from build123d import *

# Parameters (mm, degrees)
SKETCH2_W                      = 500
SKETCH2_H                      = 30
BOSS_EXTRUDE1_DEPTH            = 10
CONVERT_SOLID1_START           = -500
CONVERT_SOLID1_DEPTH           = 497
CONVERT_SOLID1_START_2         = -3.414213562
CONVERT_SOLID1_2_DEPTH         = 3.414213562
CONVERT_SOLID1_START_3         = -3.5
CONVERT_SOLID1_3_DEPTH         = 0.085786438
CONVERT_SOLID1_START_4         = 290.130873959
CONVERT_SOLID1_4_DEPTH         = 23.171572876
EDGE_FLANGE1_STRIP_W           = 10
EDGE_FLANGE1_STRIP_H           = 2
EDGE_FLANGE1_STRIP_CUT_DEPTH   = 496.585786438
EDGE_FLANGE1_STRIP_2_W         = 10
EDGE_FLANGE1_STRIP_2_H         = 2
EDGE_FLANGE1_STRIP_CUT_2_DEPTH = 496.585786438
EDGE_FLANGE1_DEPTH             = 496.585786438
EDGE_FLANGE1_BEND_DEPTH        = 496.585786438
CUT_EXTRUDE1_DEPTH             = 592.923511083
CUT_EXTRUDE1_DEPTH_BACK        = 592.923511083
SKETCH43_R                     = 3


with BuildPart() as part:
    # Sketch2 → Boss-Extrude1 (new body)
    with BuildSketch(Plane.XY):
        with Locations((-250, 301.716660397)):
            Rectangle(SKETCH2_W, SKETCH2_H)
    extrude(amount=BOSS_EXTRUDE1_DEPTH)

    # Convert-Solid1: read off the stored shape, not the designer's step
    # Convert-Solid1 outline → Convert-Solid1 (cut)
    with BuildSketch(Plane.YZ.offset(CONVERT_SOLID1_START)):
        with BuildLine():
            Line((314.716660397, 3), (314.716660397, 10))
            Line((314.716660397, 10), (288.716660397, 10))
            Line((288.716660397, 10), (288.716660397, 3))
            ThreePointArc((288.716660397, 3), (289.009553616, 2.292893219), (289.716660397, 2))
            Line((289.716660397, 2), (313.716660397, 2))
            ThreePointArc((313.716660397, 2), (314.423767178, 2.292893219), (314.716660397, 3))
        make_face()
        with BuildLine():
            Line((316.716660397, 0), (316.716660397, 3))
            ThreePointArc((316.716660397, 3), (315.837980741, 0.878679656), (313.716660397, 0))
            Line((313.716660397, 0), (316.716660397, 0))
        make_face()
        with BuildLine():
            Line((286.716660397, 0), (289.716660397, 0))
            ThreePointArc((289.716660397, 0), (287.595340053, 0.878679656), (286.716660397, 3))
            Line((286.716660397, 3), (286.716660397, 0))
        make_face()
    extrude(amount=CONVERT_SOLID1_DEPTH, mode=Mode.SUBTRACT)

    # Convert-Solid1 2 outline → Convert-Solid1 2 (cut)
    with BuildSketch(Plane.YZ.offset(CONVERT_SOLID1_START_2)):
        Polygon((316.716660397, 10), (313.302446835, 10), (313.302446835, 3.5), (313.216660397, 3.5), (313.216660397, 0), (316.716660397, 0), align=None)
        Polygon((290.130873959, 3.5), (290.130873959, 10), (286.716660397, 10), (286.716660397, 0), (290.216660397, 0), (290.216660397, 3.5), align=None)
    extrude(amount=CONVERT_SOLID1_2_DEPTH, mode=Mode.SUBTRACT)

    # Convert-Solid1 3 outline → Convert-Solid1 3 (cut)
    with BuildSketch(Plane.YZ.offset(CONVERT_SOLID1_START_3)):
        with BuildLine():
            Line((316.716660397, 3.5), (314.716660397, 3.5))
            Line((314.716660397, 3.5), (314.716660397, 3))
            ThreePointArc((314.716660397, 3), (314.423767178, 2.292893219), (313.716660397, 2))
            Line((313.716660397, 2), (313.216660397, 2))
            Line((313.216660397, 2), (313.216660397, 0))
            Line((313.216660397, 0), (313.716660397, 0))
            ThreePointArc((313.716660397, 0), (315.837980741, 0.878679656), (316.716660397, 3))
            Line((316.716660397, 3), (316.716660397, 3.5))
        make_face()
        with BuildLine():
            Line((290.216660397, 0), (290.216660397, 2))
            Line((290.216660397, 2), (289.716660397, 2))
            ThreePointArc((289.716660397, 2), (289.009553616, 2.292893219), (288.716660397, 3))
            Line((288.716660397, 3), (288.716660397, 3.5))
            Line((288.716660397, 3.5), (286.716660397, 3.5))
            Line((286.716660397, 3.5), (286.716660397, 3))
            ThreePointArc((286.716660397, 3), (287.595340053, 0.878679656), (289.716660397, 0))
            Line((289.716660397, 0), (290.216660397, 0))
        make_face()
    extrude(amount=CONVERT_SOLID1_3_DEPTH, mode=Mode.SUBTRACT)

    # Convert-Solid1 4 outline → Convert-Solid1 4 (cut)
    with BuildSketch(Plane(origin=(0, 0, 0), x_dir=(1, 0, 0), z_dir=(0, 1, 0)).offset(CONVERT_SOLID1_START_4)):
        with BuildLine():
            ThreePointArc((-3, 0), (-0.878679656, -0.878679656), (0, -3))
            Line((0, -3), (0, 0))
            Line((0, 0), (-3, 0))
        make_face()
        with BuildLine():
            Line((-3, -2), (-3, -10))
            Line((-3, -10), (-2, -10))
            Line((-2, -10), (-2, -3))
            ThreePointArc((-2, -3), (-2.292893219, -2.292893219), (-3, -2))
        make_face()
    extrude(amount=CONVERT_SOLID1_4_DEPTH, mode=Mode.SUBTRACT)

    # Edge-Flange1: sheet metal written as solids
    # Edge-Flange1 strip (on a plane across the edge) → Edge-Flange1 strip cut (cut)
    with BuildSketch(Plane(origin=(-3.414213562, 314.716660397, 10), x_dir=(0, 0, -1), z_dir=(-1, 0, 0))):
        with Locations((-2, -1)):
            Rectangle(EDGE_FLANGE1_STRIP_W, EDGE_FLANGE1_STRIP_H)
    extrude(amount=EDGE_FLANGE1_STRIP_CUT_DEPTH, mode=Mode.SUBTRACT)

    # Edge-Flange1 strip 2 (on a plane across the edge) → Edge-Flange1 strip cut 2 (cut)
    with BuildSketch(Plane(origin=(-500, 288.716660397, 10), x_dir=(0, 0, -1), z_dir=(1, 0, 0))):
        with Locations((-2, -1)):
            Rectangle(EDGE_FLANGE1_STRIP_2_W, EDGE_FLANGE1_STRIP_2_H)
    extrude(amount=EDGE_FLANGE1_STRIP_CUT_2_DEPTH, mode=Mode.SUBTRACT)

    # Edge-Flange1 section (on a plane across the edge) → Edge-Flange1 (add)
    with BuildSketch(Plane(origin=(-3.414213562, 314.716660397, 10), x_dir=(0, 0, -1), z_dir=(-1, 0, 0))):
        with BuildLine():
            Line((0, 1), (0, 3))
            Line((0, 3), (2, 3))
            Line((2, 3), (2, 1))
            ThreePointArc((2, 1), (2.292893219, 0.292893219), (3, 0))
            Line((3, 0), (3, -2))
            ThreePointArc((3, -2), (0.878679656, -1.121320344), (0, 1))
        make_face()
    extrude(amount=EDGE_FLANGE1_DEPTH)

    # Edge-Flange1 section 2 (on a plane across the edge) → Edge-Flange1 bend (add)
    with BuildSketch(Plane(origin=(-500, 288.716660397, 10), x_dir=(0, 0, -1), z_dir=(1, 0, 0))):
        with BuildLine():
            Line((0, 1), (0, 3))
            Line((0, 3), (2, 3))
            Line((2, 3), (2, 1))
            ThreePointArc((2, 1), (2.292893219, 0.292893219), (3, 0))
            Line((3, 0), (3, -2))
            ThreePointArc((3, -2), (0.878679656, -1.121320344), (0, 1))
        make_face()
    extrude(amount=EDGE_FLANGE1_BEND_DEPTH)

    # Sketch43 → Cut-Extrude1 (cut, two sides: drawn at the far end of the back side and taken through both)
    with BuildSketch(Plane.XY.offset(2).offset(-CUT_EXTRUDE1_DEPTH_BACK)):
        with Locations((-63, 301.726660397)):
            Circle(SKETCH43_R)
        with Locations((-13, 301.726660397)):
            Circle(SKETCH43_R)
        with Locations((-133, 301.726660397)):
            Circle(SKETCH43_R)
        with Locations((-83, 301.726660397)):
            Circle(SKETCH43_R)
        with Locations((-203, 301.726660397)):
            Circle(SKETCH43_R)
        with Locations((-153, 301.726660397)):
            Circle(SKETCH43_R)
        with Locations((-273, 301.726660397)):
            Circle(SKETCH43_R)
        with Locations((-223, 301.726660397)):
            Circle(SKETCH43_R)
        with Locations((-343, 301.726660397)):
            Circle(SKETCH43_R)
        with Locations((-293, 301.726660397)):
            Circle(SKETCH43_R)
        with Locations((-413, 301.726660397)):
            Circle(SKETCH43_R)
        with Locations((-363, 301.726660397)):
            Circle(SKETCH43_R)
        with Locations((-483, 301.726660397)):
            Circle(SKETCH43_R)
        with Locations((-433, 301.726660397)):
            Circle(SKETCH43_R)
        with BuildLine():
            Line((-25.99, 304.726660397), (-50.01, 304.726660397))
            ThreePointArc((-50.01, 304.726660397), (-52.124249276, 303.850909673), (-53, 301.736660397))
            Line((-53, 301.736660397), (-53, 301.716660397))
            ThreePointArc((-53, 301.716660397), (-52.124249276, 299.602411121), (-50.01, 298.726660397))
            Line((-50.01, 298.726660397), (-25.99, 298.726660397))
            ThreePointArc((-25.99, 298.726660397), (-23.875750724, 299.602411121), (-23, 301.716660397))
            Line((-23, 301.716660397), (-23, 301.736660397))
            ThreePointArc((-23, 301.736660397), (-23.875750724, 303.850909673), (-25.99, 304.726660397))
        make_face()
        with BuildLine():
            Line((-93, 301.736660397), (-93, 301.716660397))
            ThreePointArc((-93, 301.716660397), (-93.875750724, 299.602411121), (-95.99, 298.726660397))
            Line((-95.99, 298.726660397), (-120.01, 298.726660397))
            ThreePointArc((-120.01, 298.726660397), (-122.124249276, 299.602411121), (-123, 301.716660397))
            Line((-123, 301.716660397), (-123, 301.736660397))
            ThreePointArc((-123, 301.736660397), (-122.124249276, 303.850909673), (-120.01, 304.726660397))
            Line((-120.01, 304.726660397), (-95.99, 304.726660397))
            ThreePointArc((-95.99, 304.726660397), (-93.875750724, 303.850909673), (-93, 301.736660397))
        make_face()
        with BuildLine():
            Line((-163, 301.736660397), (-163, 301.716660397))
            ThreePointArc((-163, 301.716660397), (-163.875750724, 299.602411121), (-165.99, 298.726660397))
            Line((-165.99, 298.726660397), (-190.01, 298.726660397))
            ThreePointArc((-190.01, 298.726660397), (-192.124249276, 299.602411121), (-193, 301.716660397))
            Line((-193, 301.716660397), (-193, 301.736660397))
            ThreePointArc((-193, 301.736660397), (-192.124249276, 303.850909673), (-190.01, 304.726660397))
            Line((-190.01, 304.726660397), (-165.99, 304.726660397))
            ThreePointArc((-165.99, 304.726660397), (-163.875750724, 303.850909673), (-163, 301.736660397))
        make_face()
        with BuildLine():
            Line((-233, 301.736660397), (-233, 301.716660397))
            ThreePointArc((-233, 301.716660397), (-233.875750724, 299.602411121), (-235.99, 298.726660397))
            Line((-235.99, 298.726660397), (-260.01, 298.726660397))
            ThreePointArc((-260.01, 298.726660397), (-262.124249276, 299.602411121), (-263, 301.716660397))
            Line((-263, 301.716660397), (-263, 301.736660397))
            ThreePointArc((-263, 301.736660397), (-262.124249276, 303.850909673), (-260.01, 304.726660397))
            Line((-260.01, 304.726660397), (-235.99, 304.726660397))
            ThreePointArc((-235.99, 304.726660397), (-233.875750724, 303.850909673), (-233, 301.736660397))
        make_face()
        with BuildLine():
            Line((-303, 301.736660397), (-303, 301.716660397))
            ThreePointArc((-303, 301.716660397), (-303.875750724, 299.602411121), (-305.99, 298.726660397))
            Line((-305.99, 298.726660397), (-330.01, 298.726660397))
            ThreePointArc((-330.01, 298.726660397), (-332.124249276, 299.602411121), (-333, 301.716660397))
            Line((-333, 301.716660397), (-333, 301.736660397))
            ThreePointArc((-333, 301.736660397), (-332.124249276, 303.850909673), (-330.01, 304.726660397))
            Line((-330.01, 304.726660397), (-305.99, 304.726660397))
            ThreePointArc((-305.99, 304.726660397), (-303.875750724, 303.850909673), (-303, 301.736660397))
        make_face()
        with BuildLine():
            Line((-373, 301.736660397), (-373, 301.716660397))
            ThreePointArc((-373, 301.716660397), (-373.875750724, 299.602411121), (-375.99, 298.726660397))
            Line((-375.99, 298.726660397), (-400.01, 298.726660397))
            ThreePointArc((-400.01, 298.726660397), (-402.124249276, 299.602411121), (-403, 301.716660397))
            Line((-403, 301.716660397), (-403, 301.736660397))
            ThreePointArc((-403, 301.736660397), (-402.124249276, 303.850909673), (-400.01, 304.726660397))
            Line((-400.01, 304.726660397), (-375.99, 304.726660397))
            ThreePointArc((-375.99, 304.726660397), (-373.875750724, 303.850909673), (-373, 301.736660397))
        make_face()
        with BuildLine():
            Line((-443, 301.736660397), (-443, 301.716660397))
            ThreePointArc((-443, 301.716660397), (-443.875750724, 299.602411121), (-445.99, 298.726660397))
            Line((-445.99, 298.726660397), (-470.01, 298.726660397))
            ThreePointArc((-470.01, 298.726660397), (-472.124249276, 299.602411121), (-473, 301.716660397))
            Line((-473, 301.716660397), (-473, 301.736660397))
            ThreePointArc((-473, 301.736660397), (-472.124249276, 303.850909673), (-470.01, 304.726660397))
            Line((-470.01, 304.726660397), (-445.99, 304.726660397))
            ThreePointArc((-445.99, 304.726660397), (-443.875750724, 303.850909673), (-443, 301.736660397))
        make_face()
    extrude(amount=CUT_EXTRUDE1_DEPTH + CUT_EXTRUDE1_DEPTH_BACK, mode=Mode.SUBTRACT)


solid = part.part
CAD build for the part. Positions are in the model's coordinates, mm. Coordinates: 2 decimals unless noted, no trailing zeros. Write each loop counter-clockwise with the first axis right and the second up, starting at its lowest first coordinate (ties: lowest second). Pieces come first, ordered by that corner, then holes. Notation, with made-up numbers: (72, -2.5) - (126, -2.5) arc R18 ccw to (126, 30.5) - close; hole circle Ø6 at (76, 55). An arc over 180 degrees is marked (long way). Use a Markdown table: item, result. Add a question column.
Item 1: Band-saw the part on A-A, the plane x = -181. Give the cut face in (y, z), and give its area (3 significant figures).
Item 2: Flat gauge pins, fed straight in: pin 1 (8 mm diameter, centred on x = -146.5, y = 298.5, fed in from +Z); pin 2 (1 mm diameter, centred on x = -181, z = 1.5, fed in from +Y); pin 3 (1 mm diameter, centred on x = -83, z = 8, fed in from +Y); pin 4 (3 mm diameter, centred on y = 297.5, z = 2, fed in from +X). Where does each tip first touch, or does it go through?
Item 3: Drill centre lines: L1, parallel to Z at x = -357, y = 312.5; L2, parallel to Y at x = -304.5, z = 6.25; L3, parallel to Z at x = -59.5, y = 307.5. Where is each one in solid material? Low to high. Write a range as from..to.
Item 4: Mould opens along Y. For faces 1 (the face through (-500, 301.9, 1.6)), 2 (the face through (-255, 296, 2)) say: pulls with the +Y half, pulls with the -Y half, needs draft (parallel to the pull), parting line crosses it, or undercut.
Numbers:
| question | item | result |
|---|---|---|
| 1 | outline | (286.72, 3) arc R3 ccw to (289.72, 0) - (298.73, 0) - (298.73, 2) - (289.72, 2) arc R1 cw to (288.72, 3) - (288.72, 7) arc R1 cw to (289.72, 8) - (291.72, 8) - (291.72, 10) - (289.72, 10) arc R3 ccw to (286.72, 7) - close; (304.73, 0) - (313.72, 0) arc R3 ccw to (316.72, 3) - (316.72, 7) arc R3 ccw to (313.72, 10) - (311.72, 10) - (311.72, 8) - (313.72, 8) arc R1 cw to (314.72, 7) - (314.72, 3) arc R1 cw to (313.72, 2) - (304.73, 2) - close |
| 1 | area | 85.1 mm2 |
| 2 | pin 1 | z = 2 |
| 2 | pin 2 | y = 316.55 |
| 2 | pin 3 | y = 316.67 |
| 2 | pin 4 | x = 0 |
| 3 | L1 | 0..2, 8..10 |
| 3 | L2 | 286.72..288.72, 314.72..316.72 |
| 3 | L3 | 0..2 |
| 4 | face 1 | needs draft |
| 4 | face 2 | undercut |
